For this review, take the finished solid that the model builds, in its own axes (mm). A direction names the side the tool comes from. Round coordinates to 2 decimals unless told otherwise and drop trailing zeros. Order: outer loops, then holes, each group sorted by start corner. A loop starts at its lowest first (then second) coordinate and runs counter-clockwise, first axis right, second up.
Autodesk Inventor part; units mm, degrees
ref_plane "YZ Plane" through (0, 0, 0) normal (1, 0, 0) x (0, 1, 0)
ref_plane "XZ Plane" through (0, 0, 0) normal (0, 1, 0) x (-1, 0, 0)
ref_plane "XY Plane" through (0, 0, 0) normal (0, 0, 1) x (1, 0, 0)
sketch "Sketch1" plane through (0, 0, 0) normal (0, 0, 1) x (1, 0, 0)
  line L0 (135, -80) -> (-135, -80)
  line L1 (-135, -80) -> (-135, 80)
  line L2 (-135, 80) -> (135, 80)
  line L3 (135, 80) -> (135, -80)
  line L4 (135, -80) -> (-135, 80) construction
  line L5 (-135, -80) -> (135, 80) construction
  point P0 (0, 0)
  dimension "d0" = 270
  dimension "d1" = 160
extrude "Extrusion1" add sketch "Sketch1" along normal blind 10
sketch "Sketch2" plane through (0, 0, 10) normal (0, 0, 1) x (1, 0, 0)
  line L0 (70, -60) -> (-70, -60) construction
  line L1 (-70, -60) -> (-70, 60) construction
  line L2 (-70, 60) -> (70, 60) construction
  line L3 (70, 60) -> (70, -60) construction
  line L4 (70, -60) -> (-70, 60) construction
  line L5 (-70, -60) -> (70, 60) construction
  point P0 (0, 0)
  dimension "d4" = 140
  dimension "d5" = 120
hole "Hole1" at (-70, 60, 10) at (70, 60, 10) at (-70, -60, 10) at (70, -60, 10) direction (0, 0, -1) diameter 4.917 depth 25 tip angle 118
sketch "Sketch3" plane through (0, 0, 0) normal (0, 0, -1) x (-1, 0, 0)
  line L0 (135, 80) -> (135, -80) construction
  line L1 (135, -80) -> (105, -80) construction
  line L2 (105, -80) -> (105, -20) construction
  line L3 (105, -20) -> (135, -20) construction
  line L4 (135, -20) -> (135, -80) construction
  line L5 (135, 80) -> (85, 80)
  line L6 (85, 80) -> (85, -5)
  line L7 (85, -5) -> (135, -5)
  line L8 (135, -5) -> (135, 80)
  point P0 (0, 0)
  dimension "d15" = 30
  dimension "d16" = 60
  dimension "d17" = 50
  dimension "d21" = 85
extrude "Extrusion2" cut sketch "Sketch3" against normal blind 10
fillet "Fillet2" radius 15 3 edges at (-85, 80, 5) (-85, -5, 5) (-135, -5, 5)
mirror "Mirror1" about plane through (0, 0, 0) normal (1, 0, 0) of "Extrusion2"
mirror "Mirror2" about plane through (0, 0, 0) normal (1, 0, 0) of "Fillet2"
sketch "Sketch4" plane through (0, 0, 0) normal (0, 0, -1) x (-1, 0, 0)
  line L0 (-130, -32) -> (-110, -32) construction
  line L1 (-110, -32) -> (-110, -62) construction
  line L2 (-110, -62) -> (-130, -62) construction
  line L3 (-130, -62) -> (-130, -32) construction
  line L4 (135, -80) -> (-135, -80) construction
  line L5 (-135, -80) -> (-135, -20) construction
  point P0 (0, 0)
  point P1 (-120, -62)
  point P2 (-130, -47)
  dimension "d22" = 20
  dimension "d23" = 30
  dimension "d24" = 18
  dimension "d25" = 5
hole "Hole2" at (130, -32, 0) at (110, -32, 0) at (110, -62, 0) at (130, -62, 0) direction (0, 0, 1) diameter 4.134 end through all
sketch "Sketch5" plane through (-135, -80, 0) normal (0, -1, 0) x (1, 0, 0)
  line L0 (270, 0) -> (270, 10)
  line L1 (0, 0) -> (270, 0)
  point P0 (135, 0)
  point P1 (255, 5)
  point P2 (270, 5)
  dimension "d33" = 15
  dimension "d34" = 5
hole "Hole3" at (120, -80, 5) direction (0, 1, 0) diameter 4.917 depth 15 tip angle 118
mirror "Mirror3" about plane through (0, 0, 0) normal (1, 0, 0) of "Hole2", "Hole3"
chamfer "Chamfer2" distance 2 angle 45 13 edges at (-80.6066, 75.6066, 0) (-85, 37.5, 0) (-89.3934, -0.6066, 0) (-110, -5, 0) (-130.6066, -9.3934, 0) (-135, -50, 0) (0, 80, 0) (80.6066, 75.6066, 0) (85, 37.5, 0) (89.3934, -0.6066, 0) (110, -5, 0) (130.6066, -9.3934, 0) (135, -50, 0)
properties part number "Support_lift" material "Stainless Steel"
(1) Wall thickness on L1, parallel to X at y = -32, z = 6; L2, parallel to Y at x = -70, z = 5.25; L3, parallel to Y at x = 110, z = 3: over which ranges is each line inside the solid? List them lowest first.
(2) Add section A-A on y = 32.5. Give the boundary of the cut face in (x, z).
(3) Draft analysis for pull direction Z (two halves, no side actions). For faces 1 (the face through (-2, -17, 10)), 2 (the face through (-120.38, -63.78, 4.8)), 3 (the face through (89.28, -0.49, 6.06)), state which applies: pulls with the +Z half, pulls with the -Z half, needs draft (parallel to the pull), parting line crosses it, or undercut.
(4) Clearance check with flat-ended pins moving along their axes: P1, Ø6, axis at y = 62.5, z = 4, coming from the +X side; P2, Ø1, axis at x = -60.5, y = 51.5, coming from the -Z side; P3, Ø4, axis at x = -112.5, z = 6, coming from the +Y side; P4, Ø4, axis at y = 27.5, z = 7.5, coming from the -X side. State where each tip first meets the part, or that it passes through.
(5) Tool access review of faces 4 (the face through (110, -5, 6)), 5 (the face through (-2, -17, 0)), 6 (the face through (-110, -5, 6)): name each direction out of +Z, -Z, +X, -X, +Y, -Y from which nothing blocks a thin tool from reaching the whole face with its end or side.
Here are the results:
1. L1: x = -135 to -132.07, -127.93 to -112.07, -107.93 to 107.93, 112.07 to 127.93, 132.07 to 135
1. L2: y = -80 to -62.46, -57.54 to 57.54, 62.46 to 80
1. L3: y = -80 to -64.07, -59.93 to -34.07, -29.93 to -5
2. outline: (-85, 2) - (-83, 0) - (83, 0) - (85, 2) - (85, 10) - (-85, 10) - close
3. face 1: pulls with the +Z half
3. face 2: undercut
3. face 3: needs draft
4. P1: stops at x = 85
4. P2: stops at z = 0
4. P3: stops at y = -5
4. P4: stops at x = -85
5. face 4: +Z, -Z, +X, +Y
5. face 5: -Z, +X, -X, +Y, -Y
5. face 6: +Z, -Z, -X, +Y
